```python
from build123d import *

# Parameters (mm, degrees)
ESQUISSE1_R                                = 30
BOSS_EXTRU_1_DEPTH                         = 15
ESQUISSE2_R                                = 12.5
BOSS_EXTRU_2_DEPTH                         = 124
ESQUISSE4_2_W                              = 230
ESQUISSE4_2_H                              = 40
ENL_V_MAT_EXTRU_1_DEPTH                    = 5
CHAMBRAGE_POUR_VIS_T_TE_HEXAGONALE_2_COUNT = 2
CHAMBRAGE_POUR_VIS_T_TE_HEXAGONALE_2_PITCH = 41
ESQUISSE17_R                               = 6
BOSS_EXTRU_4_DEPTH                         = 83.38
ESQUISSE18_W                               = 10.356322474
ESQUISSE18_H                               = 3
ENL_V_MAT_EXTRU_2_DEPTH                    = 3
ESQUISSE19_W                               = 7.933443835
ESQUISSE19_H                               = 21.9317122
ENL_V_MAT_EXTRU_3_DEPTH                    = 50
BOSS_EXTRU_6_START                         = -10
ESQUISSE21_R                               = 12.5
BOSS_EXTRU_6_DEPTH                         = 10


with BuildPart() as part:
    # Esquisse1 → Boss.-Extru.1 (new body)
    with BuildSketch(Plane.XY):
        Circle(ESQUISSE1_R)
    extrude(amount=BOSS_EXTRU_1_DEPTH)

    # Esquisse2 → Boss.-Extru.2 (add)
    with BuildSketch(Plane(origin=(0, 0, 0), x_dir=(-1, 0, 0), z_dir=(0, 0, -1))):
        with Locations(Location((0, 0, 0), (0, 0, 180))):
            Circle(ESQUISSE2_R)
    extrude(amount=BOSS_EXTRU_2_DEPTH)

    # Esquisse4_2 → Enl_v. mat.-Extru.1 (cut)
    with BuildSketch(Plane.XY.offset(15)):
        Rectangle(ESQUISSE4_2_W, ESQUISSE4_2_H)
    extrude(amount=-ENL_V_MAT_EXTRU_1_DEPTH, mode=Mode.SUBTRACT)

    # Esquisse14 → Chambrage pour vis _ t_te hexagonale M51 (revolve, cut)
    with BuildSketch(Plane.YZ.offset(-20.5)):
        Polygon((0, 0), (0, 15), (2.75, 15), (2.75, 3.605), (2.775, 3.58), (6.12, 3.58), (6.12, 0), align=None)
    chambrage_pour_vis_t_te_hexagonale_m51 = revolve(axis=Axis((-20.5, 0, -6.35), (0, 0, 1)), mode=Mode.SUBTRACT)

    # Chambrage pour vis _ t_te hexagonale 2: Chambrage pour vis _ t_te hexagonale M51 ×2
    with Locations(*[(i * CHAMBRAGE_POUR_VIS_T_TE_HEXAGONALE_2_PITCH, 0, 0) for i in range(1, CHAMBRAGE_POUR_VIS_T_TE_HEXAGONALE_2_COUNT)]):
        add(chambrage_pour_vis_t_te_hexagonale_m51, mode=Mode.SUBTRACT)

    # Esquisse17 → Boss.-Extru.4 (add)
    with BuildSketch(Plane(origin=(0, 0, -124), x_dir=(-1, 0, 0), z_dir=(0, 0, -1))):
        Circle(ESQUISSE17_R)
    extrude(amount=BOSS_EXTRU_4_DEPTH)

    # Esquisse18 → Enl_v. mat.-Extru.2 (cut)
    with BuildSketch(Plane(origin=(0, 0, -207.38), x_dir=(-1, 0, 0), z_dir=(0, 0, -1))):
        with Locations((1.787207702, 0)):
            Rectangle(ESQUISSE18_W, ESQUISSE18_H)
    extrude(amount=-ENL_V_MAT_EXTRU_2_DEPTH, mode=Mode.SUBTRACT)

    # Esquisse19 → Enl_v. mat.-Extru.3 (cut)
    with BuildSketch(Plane(origin=(0, 0, -124), x_dir=(-1, 0, 0), z_dir=(0, 0, -1))):
        with Locations((9.966721917, 0)):
            Rectangle(ESQUISSE19_W, ESQUISSE19_H)
    extrude(amount=-ENL_V_MAT_EXTRU_3_DEPTH, mode=Mode.SUBTRACT)

    # Esquisse21 → Boss.-Extru.6 (add)
    with BuildSketch(Plane(origin=(0, 0, -124), x_dir=(-1, 0, 0), z_dir=(0, 0, -1)).offset(BOSS_EXTRU_6_START)):
        with Locations(Location((0, 0, 0), (0, 0, 180))):
            Circle(ESQUISSE21_R)
    extrude(amount=BOSS_EXTRU_6_DEPTH)


solid = part.part
```
For this review, take the finished solid that the model builds, in its own axes (mm). A direction names the side the tool comes from. Round coordinates to 2 decimals unless told otherwise and drop trailing zeros. Write each loop counter-clockwise with the first axis right and the second up, starting at its lowest first coordinate (ties: lowest second). Pieces come first, ordered by that corner, then holes. Notation, with made-up numbers: (30, 36.25) -> (83, 36.25) arc R19 ccw to (83, 72.25) -> close; hole circle Ø11 at (50, 52). An arc over 180 degrees is marked (long way). One line per question, with ' | ' between items. Start each with the question number.
(1) Add section D-D, the plane z = -71. Write out the cut boundary in (x, y), plus the area to 3 significant figures.
(2) Mouldability with a two-part tool opening along Y and no side actions: class faces 1 (the face through (-3.905, 29.745, 5.728)), 2 (the face through (22, -3, 3.58)), 3 (the face through (-9, 0, -114)) as released by +Y, released by -Y, zero draft, split by the parting line, or undercut.
(3) Add section C-C, the plane y = 26. Write out the cut boundary in (x, z), plus the area to 3 significant figures.
(4) Add section B-B, the plane z = -165.5. Write out the cut boundary in (x, y), plus the area to 3 significant figures.
(5) Add section A-A, the plane x = 0. Write out the cut boundary in (y, z), plus the area to 3 significant figures.
(6) For line 1 along X through (y, z) = (0, 6.75); line 2 along X through (y, z) = (0, 2); line 3 along Y through (x, z) = (20, 2), list the stretches that pass through material, from the lowest coordinate up. Write a range as from..to.
(7) Tool access review of faces 4 (the face through (0, -3, -207.38)), 5 (the face through (-8, 0, -74)), 6 (the face through (0, 20, 13)), 7 (the face through (0, -24, 15)), 8 (the face through (-19, -3, 3.58)): name each direction out of +Z, -Z, +X, -X, +Y, -Y from which nothing blocks a thin tool from reaching the whole face with its end or side.
(8) Insertion check: P1, Ø1.5, axis at x = 1.5, z = 12, coming from the -Y side; P2, Ø4, axis at x = 14, y = -6.5, coming from the +Z side; P3, Ø6, axis at y = 8.5, z = -12, coming from the -X side (3 decimals); P4, Ø2, axis at x = -14, z = -126, coming from the -Y side. Each pin has a flat end and moves straight along its axis. Give the tip position at first contact, or say it passes through.
Answer list:
1) outline: circle Ø25 at (0, 0) | area: 491 mm²
2) face 1: split by the parting line | face 2: undercut | face 3: zero draft
3) outline: (-14.97, 0) -> (14.97, 0) -> (14.97, 15) -> (-14.97, 15) -> close | area: 449 mm²
4) outline: circle Ø12 at (0, 0) | area: 113 mm²
5) outline: (-30, 0) -> (-12.5, 0) -> (-12.5, -124) -> (-6, -124) -> (-6, -207.38) -> (-1.5, -207.38) -> (-1.5, -204.38) -> (1.5, -204.38) -> (1.5, -207.38) -> (6, -207.38) -> (6, -124) -> (12.5, -124) -> (12.5, 0) -> (30, 0) -> (30, 15) -> (20, 15) -> (20, 10) -> (-20, 10) -> (-20, 15) -> (-30, 15) -> close | area: 4,790 mm²
6) line 1: -30..-23.25, -17.75..17.75, 23.25..30 | line 2: -30..-26.62, -14.38..14.38, 26.62..30 | line 3: -22.36..-6.1, 6.1..22.36
7) face 4: -Z, +X, -X, +Y, -Y | face 5: -X, +Y, -Y | face 6: +Z, +X, -X | face 7: +Z, +X, -X, +Y, -Y | face 8: -Z
8) P1: y = -29.99 | P2: z = 10 | P3: x = -11.225 | P4: through
